Autodesk Inventor part; units mm, degrees
ref_plane "YZ Plane" through (0, 0, 0) normal (1, 0, 0) x (0, 1, 0)
ref_plane "XZ Plane" through (0, 0, 0) normal (0, 1, 0) x (-1, 0, 0)
ref_plane "XY Plane" through (0, 0, 0) normal (0, 0, 1) x (1, 0, 0)
sketch "Sketch1" plane through (0, 0, 0) normal (0, 1, 0) x (-1, 0, 0)
  line L0 (125, 90) -> (-125, 90)
  line L1 (-125, 90) -> (-125, -90)
  line L2 (-125, -90) -> (125, -90)
  line L3 (125, -90) -> (125, 90)
  line L4 (125, 90) -> (-125, -90) construction
  line L5 (-125, 90) -> (125, -90) construction
  line L6 (0, 90) -> (80, 90)
  line L7 (80, 90) -> (-80, 90)
  line L8 (-80, 90) -> (-80, 110)
  line L9 (-80, 110) -> (80, 110)
  line L10 (80, 110) -> (80, 90)
  line L11 (80, -90) -> (-80, -90)
  line L12 (-80, -90) -> (-80, -110)
  line L13 (-80, -110) -> (80, -110)
  line L14 (80, -110) -> (80, -90)
  line L15 (0, 0) -> (0, -104)
  line L16 (0, -104) -> (0, -107)
  circle A0 centre (0, -107) radius 1.5
  line L17 (0, -107) -> (60, -107)
  line L18 (0, -107) -> (-60, -107)
  circle A1 centre (60, -107) radius 1.5
  circle A2 centre (-60, -107) radius 1.5
  line L19 (0, 0) -> (20.0042, 0)
  circle A3 centre (0, 107) radius 1.5
  circle A4 centre (60, 107) radius 1.5
  circle A5 centre (-60, 107) radius 1.5
  dimension "d0" = 250
  dimension "d1" = 180
  dimension "d2" = 80
  dimension "d3" = 160
  dimension "d4" = 20
  dimension "d5" = 160
  dimension "d6" = 20
  dimension "d7" = 104
  dimension "d8" = 3
  dimension "d9" = 3
  dimension "d10" = 60
  dimension "d11" = 60
  dimension "d12" = 3
  dimension "d13" = 3
extrude "Extrusion1" add sketch "Sketch1" along normal blind 1.5
properties part number "basePlate"
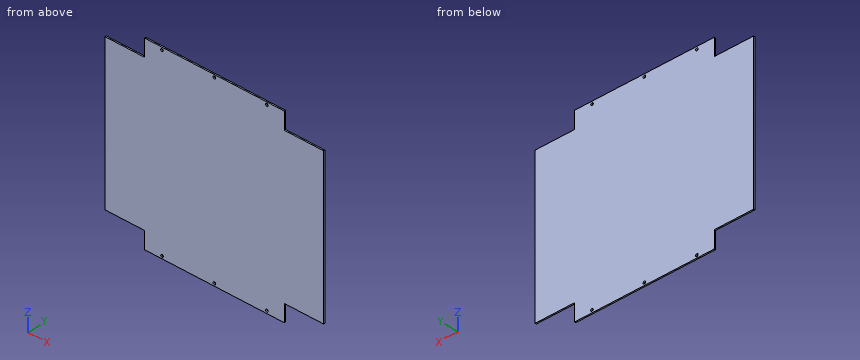
For this review, take the finished solid that the model builds, in its own axes (mm). Give positions to 0.01 mm unless a question says otherwise; leave off trailing zeros. Loops run counter-clockwise (first coordinate to the right, second up) from the corner with the lowest first, then second, coordinate; pieces in that order, holes last.
Item 1: Insertion check: pin 1 (0.8 mm diameter, centred on y = 0.5, z = 96, fed in from -X); pin 2 (2.5 mm diameter, centred on x = 0, z = -107, fed in from -Y); pin 3 (0.8 mm diameter, centred on y = 1, z = -97.5, fed in from +X). Each pin has a flat end and moves straight along its axis. Give the tip position at first contact, or say it passes through.
Item 2: Take a section at A-A, the plane y = 0.5. State the section outline as (x, z) points.
Item 3: For line 1 along X through (y, z) = (1.2, 107); line 2 along Z through (x, y) = (-60, 0.5); line 3 along Z through (x, y) = (-104, 0.45), list the stretches that pass through material, from the lowest coordinate up.
Calculated:
1. pin 1: stops at x = -80
1. pin 2: passes through
1. pin 3: stops at x = 80
2. outline: (-125, -90) - (-80, -90) - (-80, -110) - (80, -110) - (80, -90) - (125, -90) - (125, 90) - (80, 90) - (80, 110) - (-80, 110) - (-80, 90) - (-125, 90) - close; hole circle Ø3 at (-60, -107); hole circle Ø3 at (-60, 107); hole circle Ø3 at (0, -107); hole circle Ø3 at (0, 107); hole circle Ø3 at (60, -107); hole circle Ø3 at (60, 107)
3. line 1: x = -80 to -61.5, -58.5 to -1.5, 1.5 to 58.5, 61.5 to 80
3. line 2: z = -110 to -108.5, -105.5 to 105.5, 108.5 to 110
3. line 3: z = -90 to 90
